For this review, take the finished solid that the model builds, in its own axes (mm). Face numbers are marked on the shaded views. Coordinates: 2 decimals unless noted, no trailing zeros. Write each loop counter-clockwise with the first axis right and the second up, starting at its lowest first coordinate (ties: lowest second). Pieces come first, ordered by that corner, then holes.
```python
from build123d import *

# Parameters (mm, degrees)
CYLINDER_R         = 14.1
CYLINDER_DEPTH     = 25
PAD_DEPTH          = 20
POLARPATTERN_COUNT = 8


with BuildPart() as part:
    # Cylinder → Cylinder (join)
    with BuildSketch(Plane.XY):
        Circle(CYLINDER_R)
    extrude(amount=CYLINDER_DEPTH)

    # Sketch001 (on Face2 of Cylinder) → Pad (join)
    with BuildSketch(Plane.XY.offset(25)):
        with BuildLine():
            ThreePointArc((1.35, 14.0352235465), (0, 14.9352235465), (-1.35, 14.0352235465))
            ThreePointArc((1.35, 14.0352235465), (0, 14.1), (-1.35, 14.0352235465))
        make_face()
    pad = extrude(amount=-PAD_DEPTH)

    # PolarPattern: Pad ×8 about axis
    polarpattern_axis = Axis((0, 0, 25), (0, 0, 1))
    for i in range(1, POLARPATTERN_COUNT):
        add(pad.rotate(polarpattern_axis, i * 360 / POLARPATTERN_COUNT))


solid = part.part
```
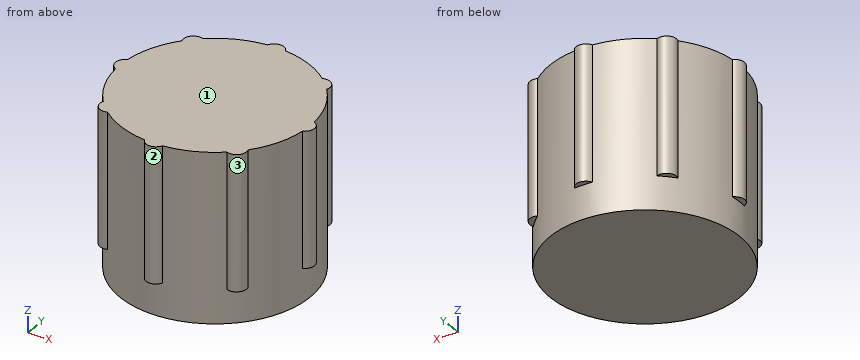
Q1. Add section C-C (y = -12.75). State the section outline as (x, z) points.
Ans:
outline: (-6.02, 0) - (6.02, 0) - (6.02, 25) - (-6.02, 25) - close
Q2. For probe 1 along Y at (x, z) = (9.5, 5.25); probe 2 along Y at (x, z) = (-9.25, 4.25); probe 3 along X at (y, z) = (7, 8), list the stretches that pass through material, from the lowest coordinate up.
Ans:
probe 1: y = -10.99 to 10.99
probe 2: y = -10.64 to 10.64
probe 3: x = -12.24 to 12.24
Q3. Add section A-A (x = 0.75). State the section outline as (y, z) points, then the cut area to 3 significant figures.
Ans:
outline: (-14.73, 5) - (-14.08, 5) - (-14.08, 0) - (14.08, 0) - (14.08, 5) - (14.73, 5) - (14.73, 25) - (-14.73, 25) - close
area: 730 mm2
Q4. Draft analysis for pull direction X (two halves, no side actions). For the marked faces 1, 2 and 3, state which applies: +X half, -X half, draft (parallel to the pull), parting line (faces both ways), or undercut.
Ans:
face 1: draft
face 2: parting line
face 3: undercut
Q5. Add section D-D (z = 4.25). State the section outline as (x, y) points.
Ans:
outline: circle Ø28.2 at (0, 0)
Q6. Clearance check with flat-ended pins moving along their axes: pin 1 Ø6 at (x, z) = (11, 19.5) entering from -Y; pin 2 Ø3 at (y, z) = (7.5, 16.5) entering from +X; pin 3 Ø1 at (x, y) = (-10, 10.5) entering from -Z; pin 4 Ø8 at (y, z) = (4.5, 11.5) entering from -X. State where each tip first meets the part, or that it passes through.
Ans:
pin 1: stops at y = -11.61
pin 2: stops at x = 12.76
pin 3: stops at z = 0
pin 4: stops at x = -14.85
